Geometry: final body of the model. Coordinates: model frame, mm. Face numbers are marked on the shaded views. Give positions to 0.01 mm unless a question says otherwise; leave off trailing zeros. Order: outer loops, then holes, each group sorted by start corner. A loop starts at its lowest first (then second) coordinate and runs counter-clockwise, first axis right, second up. Notation, with made-up numbers: (65, 45.5) - (75, 45.5) arc R38 ccw to (75, 83.5) - close; hole circle Ø10 at (75.5, 35.5). An arc over 180 degrees is marked (long way). Use one line per item in the form item = value.
from build123d import *

# Parameters (mm, degrees)
EXTRUDE_1_DEPTH     = 3.9
SKETCH_2_R          = 2.5
CUT_EXTRUDE_1_DEPTH = 0.6
CUT_EXTRUDE_2_DEPTH = 2.1
CUT_EXTRUDE_4_DEPTH = 1.9
FILLET_2_R          = 10


with BuildPart() as part:
    # 草图1 → 凸台-拉伸1 (new body)
    with BuildSketch(Plane.XY):
        with BuildLine():
            Line((-55, -39), (-30, -39))
            Line((-30, -39), (-15, -41))
            Line((-15, -41), (15, -41))
            Line((15, -41), (30, -39))
            Line((30, -39), (55, -39))
            ThreePointArc((55, -39), (57.828427125, -37.828427125), (59, -35))
            Line((59, -35), (59, 35))
            ThreePointArc((59, 35), (57.828427125, 37.828427125), (55, 39))
            Line((55, 39), (-55, 39))
            ThreePointArc((-55, 39), (-57.828427125, 37.828427125), (-59, 35))
            Line((-59, 35), (-59, -35))
            ThreePointArc((-59, -35), (-57.828427125, -37.828427125), (-55, -39))
        make_face()
    extrude(amount=EXTRUDE_1_DEPTH)

    # 草图2 → 切除-拉伸1 (cut)
    with BuildSketch(Plane.XY.offset(3.9)):
        with Locations((55, 35)):
            Circle(SKETCH_2_R)
        with Locations(Location((-55, 35, 0), (0, 0, 180))):
            Circle(SKETCH_2_R)
        with Locations(Location((55, -35, 0), (0, 0, 180))):
            Circle(SKETCH_2_R)
        with Locations((-55, -35)):
            Circle(SKETCH_2_R)
    extrude(amount=-CUT_EXTRUDE_1_DEPTH, mode=Mode.SUBTRACT)

    # 草图3 → 切除-拉伸2 (cut)
    with BuildSketch(Plane.XY.offset(3.3)):
        with BuildLine():
            Line((53.309526953, 38.625231148), (52.886908691, 39.531538935))
            ThreePointArc((52.886908691, 39.531538935), (58.535533906, 38.535533906), (59.531538935, 32.886908691))
            Line((59.531538935, 32.886908691), (58.625231148, 33.309526953))
            ThreePointArc((58.625231148, 33.309526953), (58.395478624, 33.940766826), (57.76423875, 33.711014302))
            ThreePointArc((57.76423875, 33.711014302), (52.843324317, 32.843324317), (53.711014302, 37.76423875))
            ThreePointArc((53.711014302, 37.76423875), (53.940766826, 38.395478624), (53.309526953, 38.625231148))
        make_face()
        with BuildLine():
            Line((-58.625231148, 33.309526953), (-59.531538935, 32.886908691))
            ThreePointArc((-59.531538935, 32.886908691), (-58.535533906, 38.535533906), (-52.886908691, 39.531538935))
            Line((-52.886908691, 39.531538935), (-53.309526953, 38.625231148))
            ThreePointArc((-53.309526953, 38.625231148), (-53.940766826, 38.395478624), (-53.711014302, 37.76423875))
            ThreePointArc((-53.711014302, 37.76423875), (-52.843324317, 32.843324317), (-57.76423875, 33.711014302))
            ThreePointArc((-57.76423875, 33.711014302), (-58.395478624, 33.940766826), (-58.625231148, 33.309526953))
        make_face()
        with BuildLine():
            Line((-53.309526953, -38.625231148), (-52.886908691, -39.531538935))
            ThreePointArc((-52.886908691, -39.531538935), (-58.535533906, -38.535533906), (-59.531538935, -32.886908691))
            Line((-59.531538935, -32.886908691), (-58.625231148, -33.309526953))
            ThreePointArc((-58.625231148, -33.309526953), (-58.395478624, -33.940766826), (-57.76423875, -33.711014302))
            ThreePointArc((-57.76423875, -33.711014302), (-52.843324317, -32.843324317), (-53.711014302, -37.76423875))
            ThreePointArc((-53.711014302, -37.76423875), (-53.940766826, -38.395478624), (-53.309526953, -38.625231148))
        make_face()
        with BuildLine():
            Line((58.625231148, -33.309526953), (59.531538935, -32.886908691))
            ThreePointArc((59.531538935, -32.886908691), (58.535533906, -38.535533906), (52.886908691, -39.531538935))
            Line((52.886908691, -39.531538935), (53.309526953, -38.625231148))
            ThreePointArc((53.309526953, -38.625231148), (53.940766826, -38.395478624), (53.711014302, -37.76423875))
            ThreePointArc((53.711014302, -37.76423875), (52.843324317, -32.843324317), (57.76423875, -33.711014302))
            ThreePointArc((57.76423875, -33.711014302), (58.395478624, -33.940766826), (58.625231148, -33.309526953))
        make_face()
    extrude(amount=-CUT_EXTRUDE_2_DEPTH, mode=Mode.SUBTRACT)

    # 草图5 → 切除-拉伸4 (cut)
    with BuildSketch(Plane(origin=(0, 0, 0), x_dir=(-1, 0, 0), z_dir=(0, 0, -1))):
        with BuildLine():
            Line((-51, 35), (-51, 39))
            Line((-51, 39), (51, 39))
            Line((51, 39), (51, 35))
            ThreePointArc((51, 35), (52.171572875, 32.171572875), (55, 31))
            Line((55, 31), (59, 31))
            Line((59, 31), (59, -31))
            Line((59, -31), (55, -31))
            ThreePointArc((55, -31), (52.171572875, -32.171572875), (51, -35))
            Line((51, -35), (51, -39))
            Line((51, -39), (30, -39))
            Line((30, -39), (15, -41))
            Line((15, -41), (-15, -41))
            Line((-15, -41), (-30, -39))
            Line((-30, -39), (-51, -39))
            Line((-51, -39), (-51, -35))
            ThreePointArc((-51, -35), (-52.171572875, -32.171572875), (-55, -31))
            Line((-55, -31), (-59, -31))
            Line((-59, -31), (-59, 31))
            Line((-59, 31), (-55, 31))
            ThreePointArc((-55, 31), (-52.171572875, 32.171572875), (-51, 35))
        make_face()
    extrude(amount=-CUT_EXTRUDE_4_DEPTH, mode=Mode.SUBTRACT)

    # 圆角2
    # the kernel refuses this fillet: 10 mm, written as the material it adds along each edge
    with BuildSketch(Plane(origin=(-59, -31, 1.9), x_dir=(0, 1, 0), z_dir=(1, 0, 0)), Plane(origin=(-51, 39, 1.9), x_dir=(1, 0, 0), z_dir=(0, -1, 0)), Plane(origin=(55, -31, 1.9), x_dir=(0, 1, 0), z_dir=(1, 0, 0)), Plane(origin=(51, 35, 1.9), x_dir=(-1, 0, 0), z_dir=(0, 1, 0)), Plane(origin=(59, 31, 1.9), x_dir=(0, -1, 0), z_dir=(-1, 0, 0)), Plane(origin=(-55, 31, 1.9), x_dir=(0, -1, 0), z_dir=(-1, 0, 0)), Plane(origin=(51, -39, 1.9), x_dir=(-1, 0, 0), z_dir=(0, 1, 0))) as fillet_2_piece_1:
        with BuildLine():
            CenterArc((5.864298765, -10), FILLET_2_R, 90, 35.904068583)
            Line((0, -1.9), (-0.117285975, -1.738))
            ThreePointArc((-0.117285975, -1.738), (-0.2, -0.95), (-0.2, 0))
            Line((-0.2, 0), (0, 0.2))
            Line((0, 0.2), (5.864298765, 0.2))
            Line((5.864298765, 0.2), (5.864298765, 0))
        make_face()
    extrude(amount=4)
    with BuildSketch(Plane(origin=(-55, -35, 1.9), x_dir=(0, 1, 0), z_dir=(-1, 0, 0))) as fillet_2_piece_2:
        with BuildLine():
            CenterArc((9.864298765, 10), FILLET_2_R, 234.095931417, 35.904068583)
            Line((4, 1.9), (3.882714025, 1.738))
            ThreePointArc((3.882714025, 1.738), (3.8, 0.95), (3.8, 0))
            Line((3.8, 0), (4, -0.2))
            Line((4, -0.2), (9.864298765, -0.2))
            Line((9.864298765, -0.2), (9.864298765, 0))
        make_face()
    revolve(axis=Axis((-55, -35, 1.9), (0, 0, -1)), revolution_arc=90)
    with BuildSketch(Plane(origin=(-55, 35, 1.9), x_dir=(1, 0, 0), z_dir=(0, 1, 0))) as fillet_2_piece_3:
        with BuildLine():
            CenterArc((9.864298765, 10), FILLET_2_R, 234.095931417, 35.904068583)
            Line((4, 1.9), (3.882714025, 1.738))
            ThreePointArc((3.882714025, 1.738), (3.8, 0.95), (3.8, 0))
            Line((3.8, 0), (4, -0.2))
            Line((4, -0.2), (9.864298765, -0.2))
            Line((9.864298765, -0.2), (9.864298765, 0))
        make_face()
    revolve(axis=Axis((-55, 35, 1.9), (0, 0, -1)), revolution_arc=90)
    with BuildSketch(Plane(origin=(55, -35, 1.9), x_dir=(-1, 0, 0), z_dir=(0, -1, 0))) as fillet_2_piece_4:
        with BuildLine():
            CenterArc((9.864298765, 10), FILLET_2_R, 234.095931417, 35.904068583)
            Line((4, 1.9), (3.882714025, 1.738))
            ThreePointArc((3.882714025, 1.738), (3.8, 0.95), (3.8, 0))
            Line((3.8, 0), (4, -0.2))
            Line((4, -0.2), (9.864298765, -0.2))
            Line((9.864298765, -0.2), (9.864298765, 0))
        make_face()
    revolve(axis=Axis((55, -35, 1.9), (0, 0, -1)), revolution_arc=90)
    with BuildSketch(Plane(origin=(-51, -35, 1.9), x_dir=(0, 0, -1), z_dir=(0, -1, 0))) as fillet_2_piece_5:
        with BuildLine():
            CenterArc((10, 5.864298765), FILLET_2_R, 180, 35.904068583)
            Line((0, 5.864298765), (-0.2, 5.864298765))
            Line((-0.2, 5.864298765), (-0.2, 0))
            Line((-0.2, 0), (0, -0.2))
            ThreePointArc((0, -0.2), (0.95, -0.2), (1.738, -0.117285975))
            Line((1.738, -0.117285975), (1.9, 0))
        make_face()
    extrude(amount=4)
    with BuildSketch(Plane(origin=(55, 35, 1.9), x_dir=(0, -1, 0), z_dir=(1, 0, 0))) as fillet_2_piece_6:
        with BuildLine():
            CenterArc((9.864298765, 10), FILLET_2_R, 234.095931417, 35.904068583)
            Line((4, 1.9), (3.882714025, 1.738))
            ThreePointArc((3.882714025, 1.738), (3.8, 0.95), (3.8, 0))
            Line((3.8, 0), (4, -0.2))
            Line((4, -0.2), (9.864298765, -0.2))
            Line((9.864298765, -0.2), (9.864298765, 0))
        make_face()
    revolve(axis=Axis((55, 35, 1.9), (0, 0, -1)), revolution_arc=90)


solid = part.part
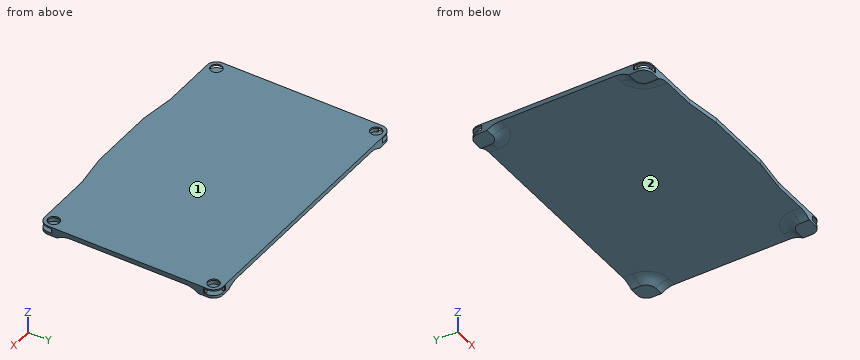
(1) Ray query, line 1 along Y through (x, z) = (55, 3.5); line 2 along Y through (x, z) = (-46.5, 2.3); line 3 along Z through (x, y) = (-29, -2.5). Return the intervals inside material, ascending.
Computed values:
line_1 = -39 to -37.5, -32.5 to 32.5, 37.5 to 39
line_2 = -39 to 39
line_3 = 1.9 to 3.9
(2) Cut plane A-A on y = -15.5. Output: boundary loops of the cut face in (x, z), plus the area to 3 significant figures.
Computed values:
outline = (-59, 1.9) - (59, 1.9) - (59, 3.9) - (-59, 3.9) - close
area = 236 mm²
(3) Cut plane C-C on z = 2.6. Output: boundary loops of the cut face in (x, y) (3 decimals).
Computed values:
outline = (-59, -33.135) - (-58.625, -33.31) arc R0.475 ccw to (-57.764, -33.711) arc R3.05 cw (long way) to (-53.711, -37.764) arc R0.475 ccw to (-53.31, -38.625) - (-53.135, -39) - (-30, -39) - (-15, -41) - (15, -41) - (30, -39) - (53.135, -39) - (53.31, -38.625) arc R0.475 ccw to (53.711, -37.764) arc R3.05 cw (long way) to (57.764, -33.711) arc R0.475 ccw to (58.625, -33.31) - (59, -33.135) - (59, 33.135) - (58.625, 33.31) arc R0.475 ccw to (57.764, 33.711) arc R3.05 cw (long way) to (53.711, 37.764) arc R0.475 ccw to (53.31, 38.625) - (53.135, 39) - (-53.135, 39) - (-53.31, 38.625) arc R0.475 ccw to (-53.711, 37.764) arc R3.05 cw (long way) to (-57.764, 33.711) arc R0.475 ccw to (-58.625, 33.31) - (-59, 33.135) - close
(4) Pull-direction query (X, two-part tool) for the marked faces 1 and 2; classes: released by +X, released by -X, zero draft, split by the parting line, or undercut.
Computed values:
face_1 = zero draft
face_2 = undercut
(5) Contact query for flat-ended pins moving along their axis: pin 1 Ø3.5 at (x, y) = (-55, -35) entering from +Z; pin 2 Ø1.5 at (x, z) = (4.5, 1) entering from +Y; pin 3 Ø1.2 at (x, z) = (-39.5, 2.5) entering from -Y. Output: stop coordinate, or through.
Computed values:
pin_1 = 1.2
pin_2 = through
pin_3 = -39
(6) Cut plane B-B on x = 41. Output: boundary loops of the cut face in (y, z), plus the area to 3 significant figures.
Computed values:
outline = (-39, 1.9) - (39, 1.9) - (39, 3.9) - (-39, 3.9) - close
area = 156 mm²
